Geometry check sheet. Reference: the model listing, model coordinates, mm. Face numbers are marked on the shaded views. A direction names the side the tool comes from. Round coordinates to 2 decimals unless told otherwise and drop trailing zeros. Order: outer loops, then holes, each group sorted by start corner. A loop starts at its lowest first (then second) coordinate and runs counter-clockwise, first axis right, second up. Notation, with made-up numbers: (70, 36) - (129, 36) arc R29 cw to (129, 66) - close; hole circle Ø10 at (50, 64). An arc over 180 degrees is marked (long way). Use a Markdown table: item, result. Add a question column.
(1) Mould release check, pull along X, two halves, no side actions. Record for the marked faces 1, 2, 3 and 4: released by +X, released by -X, zero draft, split by the parting line, or undercut.
(2) Section check D-D on x = 8. Record the boundary of the cut face in (y, z), then the cut area to 3 significant figures.
(3) Access from +Z, -Z, +X, -X, +Y, -Y to the whole of each face (thin tool, end or side, straight path). Record for the marked faces 5 and 6.
(4) Thickness scan on line 1 along X through (y, z) = (19.5, 0.5) (3 decimals); line 2 along Y through (x, z) = (-22.5, 6); line 3 along Z through (x, y) = (27.5, -26). Record the ranges inside material, lowest first. Write a range as [from, to].
(5) Section check A-A on z = 1.75. Record the boundary of the cut face in (x, y) (3 decimals), then the cut area to 3 significant figures.
(6) Gauge pin test, flat ends, axial feed: P1, Ø4.5, axis at y = -9.52, z = -2.38, coming from the +X side; P2, Ø2.5, axis at x = 15.5, z = 7.5, coming from the -Y side; P3, Ø2.5, axis at x = -12.5, z = 6.5, coming from the +Y side; P4, Ø3, axis at x = 9.5, z = 5, coming from the -Y side. Record the tip position at first contact, or that the pin passes through.
(7) Section check C-C on x = -4. Record the boundary of the cut face in (y, z), then the cut area to 3 significant figures.
(8) Section check B-B on y = 13. Record the boundary of the cut face in (x, z) (1 decimal), then the cut area to 3 significant figures.
```python
from build123d import *

# Parameters (mm, degrees)
BASE_FLANGE1_DEPTH = 38.1
CUT_EXTRUDE1_DEPTH = 2.38125
FILLET1_R          = 6.35
SKETCH7_R          = 2.413
CUT_EXTRUDE2_DEPTH = 2.38125
FILLET2_R          = 6.35


# Sheet-metal steps are written as plain solids
with BuildPart() as part:
    # Sketch1 → Base-Flange1 (new, symmetric)
    with BuildSketch(Plane(origin=(0, 0, 0), x_dir=(1, 0, 0), z_dir=(0, 1, 0))):
        with BuildLine():
            Line((-41.275, 7.9375), (-41.275, -3.175))
            ThreePointArc((-41.275, -3.175), (-39.880096045, -6.542596045), (-36.5125, -7.9375))
            Line((-36.5125, -7.9375), (36.5125, -7.9375))
            ThreePointArc((36.5125, -7.9375), (39.880096045, -6.542596045), (41.275, -3.175))
            Line((41.275, -3.175), (41.275, 7.9375))
            Line((41.275, 7.9375), (38.89375, 7.9375))
            Line((38.89375, 7.9375), (38.89375, -3.175))
            ThreePointArc((38.89375, -3.175), (38.196298023, -4.858798023), (36.5125, -5.55625))
            Line((36.5125, -5.55625), (-36.5125, -5.55625))
            ThreePointArc((-36.5125, -5.55625), (-38.196298023, -4.858798023), (-38.89375, -3.175))
            Line((-38.89375, -3.175), (-38.89375, 7.9375))
            Line((-38.89375, 7.9375), (-41.275, 7.9375))
        make_face()
    extrude(amount=BASE_FLANGE1_DEPTH, both=True)

    # Sketch6 → Cut-Extrude1 (cut)
    with BuildSketch(Plane.XY.offset(7.9375)):
        with BuildLine():
            Line((-10.540250852, 23.01875), (-1.374815329, 7.14375))
            ThreePointArc((-1.374815329, 7.14375), (0, 6.35), (1.374815329, 7.14375))
            Line((1.374815329, 7.14375), (10.540250852, 23.01875))
            ThreePointArc((10.540250852, 23.01875), (10.540250852, 24.60625), (9.165435523, 25.4))
            Line((9.165435523, 25.4), (-9.165435523, 25.4))
            ThreePointArc((-9.165435523, 25.4), (-10.540250852, 24.60625), (-10.540250852, 23.01875))
        make_face()
        with BuildLine():
            Line((14.664696837, 20.6375), (5.499261314, 4.7625))
            ThreePointArc((5.499261314, 4.7625), (5.499261314, 3.175), (6.874076643, 2.38125))
            Line((6.874076643, 2.38125), (25.204947689, 2.38125))
            ThreePointArc((25.204947689, 2.38125), (26.579763018, 3.175), (26.579763018, 4.7625))
            Line((26.579763018, 4.7625), (17.414327494, 20.6375))
            ThreePointArc((17.414327494, 20.6375), (16.039512166, 21.43125), (14.664696837, 20.6375))
        make_face()
        with BuildLine():
            Line((25.204947689, -2.38125), (6.874076643, -2.38125))
            ThreePointArc((6.874076643, -2.38125), (5.499261314, -3.175), (5.499261314, -4.7625))
            Line((5.499261314, -4.7625), (14.664696837, -20.6375))
            ThreePointArc((14.664696837, -20.6375), (16.039512166, -21.43125), (17.414327494, -20.6375))
            Line((17.414327494, -20.6375), (26.579763018, -4.7625))
            ThreePointArc((26.579763018, -4.7625), (26.579763018, -3.175), (25.204947689, -2.38125))
        make_face()
        with BuildLine():
            Line((10.540250852, -23.01875), (1.374815329, -7.14375))
            ThreePointArc((1.374815329, -7.14375), (0, -6.35), (-1.374815329, -7.14375))
            Line((-1.374815329, -7.14375), (-10.540250852, -23.01875))
            ThreePointArc((-10.540250852, -23.01875), (-10.540250852, -24.60625), (-9.165435523, -25.4))
            Line((-9.165435523, -25.4), (9.165435523, -25.4))
            ThreePointArc((9.165435523, -25.4), (10.540250852, -24.60625), (10.540250852, -23.01875))
        make_face()
        with BuildLine():
            Line((-14.664696837, -20.6375), (-5.499261314, -4.7625))
            ThreePointArc((-5.499261314, -4.7625), (-5.499261314, -3.175), (-6.874076643, -2.38125))
            Line((-6.874076643, -2.38125), (-25.204947689, -2.38125))
            ThreePointArc((-25.204947689, -2.38125), (-26.579763018, -3.175), (-26.579763018, -4.7625))
            Line((-26.579763018, -4.7625), (-17.414327494, -20.6375))
            ThreePointArc((-17.414327494, -20.6375), (-16.039512166, -21.43125), (-14.664696837, -20.6375))
        make_face()
        with BuildLine():
            Line((-25.204947689, 2.38125), (-6.874076643, 2.38125))
            ThreePointArc((-6.874076643, 2.38125), (-5.499261314, 3.175), (-5.499261314, 4.7625))
            Line((-5.499261314, 4.7625), (-14.664696837, 20.6375))
            ThreePointArc((-14.664696837, 20.6375), (-16.039512166, 21.43125), (-17.414327494, 20.6375))
            Line((-17.414327494, 20.6375), (-26.579763018, 4.7625))
            ThreePointArc((-26.579763018, 4.7625), (-26.579763018, 3.175), (-25.204947689, 2.38125))
        make_face()
        with BuildLine():
            Line((-20.622229928, 38.1), (-17.872599271, 33.3375))
            ThreePointArc((-17.872599271, 33.3375), (-15.548337957, 31.013238686), (-12.373337957, 30.1625))
            Line((-12.373337957, 30.1625), (12.373337957, 30.1625))
            ThreePointArc((12.373337957, 30.1625), (15.548337957, 31.013238686), (17.872599271, 33.3375))
            Line((17.872599271, 33.3375), (20.622229928, 38.1))
            Line((20.622229928, 38.1), (-20.622229928, 38.1))
        make_face()
        with BuildLine():
            Line((-20.622229928, -38.1), (20.622229928, -38.1))
            Line((20.622229928, -38.1), (17.872599271, -33.3375))
            ThreePointArc((17.872599271, -33.3375), (15.548337957, -31.013238686), (12.373337957, -30.1625))
            Line((12.373337957, -30.1625), (-12.373337957, -30.1625))
            ThreePointArc((-12.373337957, -30.1625), (-15.548337957, -31.013238686), (-17.872599271, -33.3375))
            Line((-17.872599271, -33.3375), (-20.622229928, -38.1))
        make_face()
    extrude(amount=-CUT_EXTRUDE1_DEPTH, mode=Mode.SUBTRACT)

    # Fillet1
    fillet1_edges = [part.edges().sort_by_distance(p)[0] for p in [
        (20.622229928, -38.1, 6.746875),
        (-20.622229928, -38.1, 6.746875),
        (-20.622229928, 38.1, 6.746875),
        (20.622229928, 38.1, 6.746875),
    ]]
    fillet(fillet1_edges, radius=FILLET1_R)

    # Sketch7 → Cut-Extrude2 (cut)
    with BuildSketch(Plane(origin=(41.275, 0, 0), x_dir=(0, 0, -1), z_dir=(1, 0, 0))):
        with Locations((2.38125, 28.575)):
            Circle(SKETCH7_R)
        with Locations((2.38125, 9.525)):
            Circle(SKETCH7_R)
        with Locations((2.38125, -9.525)):
            Circle(SKETCH7_R)
        with Locations((2.38125, -28.575)):
            Circle(SKETCH7_R)
    cut_extrude2 = extrude(amount=-CUT_EXTRUDE2_DEPTH, mode=Mode.SUBTRACT)

    # Mirror1: Cut-Extrude2 across plane
    add(cut_extrude2.mirror(Plane(origin=(0, 0, 0), x_dir=(0, 0, 1), z_dir=(1, 0, 0))), mode=Mode.SUBTRACT)

    # Fillet2
    fillet2_edges = [part.edges().sort_by_distance(p)[0] for p in [
        (40.084375, 38.1, -7.9375),
        (-40.084375, 38.1, -7.9375),
        (40.084375, -38.1, -7.9375),
        (-40.084375, -38.1, -7.9375),
    ]]
    fillet(fillet2_edges, radius=FILLET2_R)


solid = part.part
```
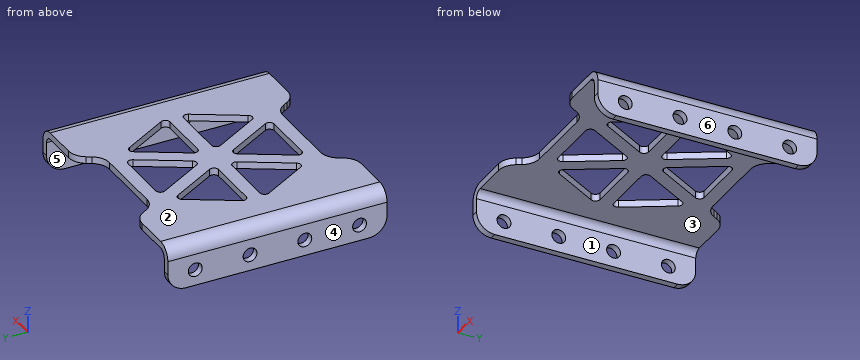
Check sheet entries:
| question | item | result |
|---|---|---|
| 1 | face 1 | undercut |
| 1 | face 2 | zero draft |
| 1 | face 3 | undercut |
| 1 | face 4 | released by -X |
| 2 | outline | (-30.16, 5.56) - (-25.4, 5.56) - (-25.4, 7.94) - (-30.16, 7.94) - close; (-18.62, 5.56) - (-9.09, 5.56) - (-9.09, 7.94) - (-18.62, 7.94) - close; (-2.38, 5.56) - (2.38, 5.56) - (2.38, 7.94) - (-2.38, 7.94) - close; (9.09, 5.56) - (18.62, 5.56) - (18.62, 7.94) - (9.09, 7.94) - close; (25.4, 5.56) - (30.16, 5.56) - (30.16, 7.94) - (25.4, 7.94) - close |
| 2 | area | 79.4 mm2 |
| 3 | face 5 | -Z, +Y, -Y |
| 3 | face 6 | +Z, -Z, +X, +Y, -Y |
| 4 | line 1 | x = [-41.275, -38.894], [38.894, 41.275] |
| 4 | line 2 | y = [-37.84, -11.83], [-2.38, 2.38], [11.83, 37.84] |
| 4 | line 3 | z = [5.56, 7.94] |
| 5 | outline | (-41.275, -38.1) - (-38.894, -38.1) - (-38.894, 38.1) - (-41.275, 38.1) - close; (38.894, -38.1) - (41.275, -38.1) - (41.275, 38.1) - (38.894, 38.1) - close |
| 5 | area | 363 mm2 |
| 6 | P1 | passes through |
| 6 | P2 | stops at y = -31.91 |
| 6 | P3 | stops at y = 30.31 |
| 6 | P4 | stops at y = -30.16 |
| 7 | outline | (-30.16, 5.56) - (-25.4, 5.56) - (-25.4, 7.94) - (-30.16, 7.94) - close; (-11.69, 5.56) - (11.69, 5.56) - (11.69, 7.94) - (-11.69, 7.94) - close; (25.4, 5.56) - (30.16, 5.56) - (30.16, 7.94) - (25.4, 7.94) - close |
| 7 | area | 78.4 mm2 |
| 8 | outline | (-41.3, -7.9) - (-38.9, -7.9) - (-38.9, 3.2) arc R2.4 cw to (-36.5, 5.6) - (-21.8, 5.6) - (-21.8, 7.9) - (-36.5, 7.9) arc R4.8 ccw to (-41.3, 3.2) - close; (-10.3, 5.6) - (-4.8, 5.6) - (-4.8, 7.9) - (-10.3, 7.9) - close; (4.8, 5.6) - (10.3, 5.6) - (10.3, 7.9) - (4.8, 7.9) - close; (21.8, 5.6) - (36.5, 5.6) arc R2.4 cw to (38.9, 3.2) - (38.9, -7.9) - (41.3, -7.9) - (41.3, 3.2) arc R4.8 ccw to (36.5, 7.9) - (21.8, 7.9) - close |
| 8 | area | 176 mm2 |
